Here's how the part is built. I have some questions about the finished solid (model axes, mm). Round coordinates to 2 decimals unless told otherwise and drop trailing zeros. Loops run counter-clockwise (first coordinate to the right, second up) from the corner with the lowest first, then second, coordinate; pieces in that order, holes last. Notation, with made-up numbers: M 63,-18.5 L 117,-18.5 A18 ccw 117,-2.5 Z; hole C 10.25,85.25 d3. An arc over 180 degrees is marked long. Use a Markdown table: item, result.
from build123d import *

# Parameters (mm, degrees)
F0_R     = 12.7
F1_DEPTH = 10
F3_DEPTH = 228.6
F4_R     = 12.7
F5_DEPTH = 10


with BuildPart() as f1:
    # F0 (on Front) → F1 (new body)
    with BuildSketch(Plane.XZ):
        Circle(F0_R)
    extrude(amount=F1_DEPTH)

    # F2 (on face) → F3 (join)
    with BuildSketch(Plane.XZ.offset(10)):
        with BuildLine():
            Line((10.6065911112, -6.985), (-10.6065911112, -6.985))
            ThreePointArc((-10.6065911112, -6.985), (0, -12.7), (10.6065911112, -6.985))
        make_face()
    extrude(amount=F3_DEPTH)

    # F4 (on face) → F5 (join)
    with BuildSketch(Plane.XZ.offset(238.6)):
        Circle(F4_R)
    extrude(amount=F5_DEPTH)


solid = f1.part
1. Imagine slicing it at C-C, the plane y = -128.5. Write out the boundary of the cut face in (x, z) (3 decimals).
Answer sheet:
| item | result |
|---|---|
| outline | M -10.607,-6.985 A12.7 ccw 10.607,-6.985 Z |
2. We'd pull the mould along Y, two halves only. Please class faces 1 (the face through (0, 0, 0)), 2 (the face through (0, -238.6, 3)), 3 (the face through (0, -248.6, 0)): +Y half, -Y half, draft (parallel to the pull), parting line (faces both ways), or undercut.
Answer sheet:
| item | result |
|---|---|
| face 1 | +Y half |
| face 2 | undercut |
| face 3 | -Y half |
3. For pin 1 Ø1 at (x, y) = (-3.5, -192) entering from -Z; pin 2 Ø6.5 at (x, y) = (0.5, -99.5) entering from +Z (3 decimals), each with a flat end and sliding along its axis, tell me the tip position at first contact or that it passes through.
Answer sheet:
| item | result |
|---|---|
| pin 1 | z = -12.34 |
| pin 2 | z = -6.985 |
4. Imagine slicing it at A-A, the plane z = 0. Write out the boundary of the cut face in (x, y).
Answer sheet:
| item | result |
|---|---|
| outline | M -12.7,-248.6 L 12.7,-248.6 L 12.7,-238.6 L -12.7,-238.6 Z; M -12.7,-10 L 12.7,-10 L 12.7,0 L -12.7,0 Z |
5. Imagine slicing it at B-B, the plane x = 0. Write out the boundary of the cut face in (y, z) (3 decimals), then the cut area to 3 significant figures.
Answer sheet:
| item | result |
|---|---|
| outline | M -248.6,-12.7 L 0,-12.7 L 0,12.7 L -10,12.7 L -10,-6.985 L -238.6,-6.985 L -238.6,12.7 L -248.6,12.7 Z |
| area | 1,810 mm2 |
6. I need wall thicknesses on probe 1 along Y at (x, z) = (10.25, 4); probe 2 along X at (y, z) = (-164, -7.75); probe 3 along Z at (x, y) = (-2.75, -138) (3 decimals). Which ranges of each line are inside material? Lowest first, please. Write a range as from..to.
Answer sheet:
| item | result |
|---|---|
| probe 1 | -248.6..-238.6, -10..0 |
| probe 2 | -10.06..10.06 |
| probe 3 | -12.399..-6.985 |
